Model file for the job. Use its own axes, mm. Give positions to 0.01 mm unless a question says otherwise; leave off trailing zeros. Write each loop counter-clockwise with the first axis right and the second up, starting at its lowest first coordinate (ties: lowest second). Pieces come first, ordered by that corner, then holes. Notation, with made-up numbers: M -7.5,43 L 28.5,43 A16 cw 28.5,67 Z; hole C -10.5,-19.5 d9. An arc over 180 degrees is marked long. Answer as a JSON object with one key per item and string values. Group by question number.
```python
from build123d import *

# Parameters (mm, degrees)
EXTRUSION1_DEPTH      = 5
TROU_TARAUD_M3X0_51_D = 3.3
TROU_TARAUD_M4X0_71_D = 3.3


with BuildPart() as part:
    # Esquisse1 → Extrusion1 (new body)
    with BuildSketch(Plane.XY):
        with BuildLine():
            Line((11.324751653, -14), (-91.324751653, -14))
            ThreePointArc((-91.324751653, -14), (-92.063300599, -13.858640755), (-92.697448823, -13.454545455))
            ThreePointArc((-92.697448823, -13.454545455), (-98.5, 0), (-92.697448823, 13.454545455))
            ThreePointArc((-92.697448823, 13.454545455), (-92.063300599, 13.858640755), (-91.324751653, 14))
            Line((-91.324751653, 14), (11.324751653, 14))
            ThreePointArc((11.324751653, 14), (12.063300599, 13.858640755), (12.697448823, 13.454545455))
            ThreePointArc((12.697448823, 13.454545455), (18.5, 0), (12.697448823, -13.454545455))
            ThreePointArc((12.697448823, -13.454545455), (12.063300599, -13.858640755), (11.324751653, -14))
        make_face()
    extrude(amount=EXTRUSION1_DEPTH)

    # Trou taraudé M3x0.51 (through all)
    with Locations(Plane.XY.offset(5)):
        with Locations((-93.6, -5), (-93.6, 5), (-45.6, -5), (-45.6, 5), (-34.4, -5), (-34.4, 5), (13.6, -5), (13.6, 5)):
            Hole(TROU_TARAUD_M3X0_51_D / 2)

    # Trou taraudé M4x0.71 (through all)
    with Locations(Plane(origin=(0, 0, 0), x_dir=(-1, 0, 0), z_dir=(0, 0, -1))):
        with Locations((0, 0)):
            Hole(TROU_TARAUD_M4X0_71_D / 2)


solid = part.part
```
Q1. Slice it at D-D, the plane x = 0.5. Write the cut outline in (y, z).
Q2. Slice it at B-B, the plane z = 2.2. Count the separate pieces of the cut face and the enclosed holes in it, then the cut area to 3 significant figures.
Q3. Slice it at A-A, the plane x = -45.6. Write the cut outline in (y, z), then the cut area to 3 significant figures.
Q4. Drop flat-ended pins along their axis: P1, Ø3, axis at x = -34.4, y = 5, coming from the +Z side; P2, Ø3, axis at y = 2, z = 2.5, coming from the -X side; P3, Ø1, axis at y = 9.5, z = 4, coming from the +X side; P4, Ø2, axis at y = -2.5, z = 1.5, coming from the -X side. Give the stop position or say it passes through.
Q5. Wall check: L1, parallel to X at y = -5.5, z = 3.6; L2, parallel to Y at x = -45.6, z = 1.6; L3, parallel to X at y = 6.5, z = 4.15. Give the ranges that are in metal, low to high.
Q6. Two-plate mould, pull along Y, no slides. Class faces 1 (the cylindrical face through (14, 3.4, 2.5)), 2 (the cylindrical face through (-98.5, -0.2, 2.5)), 3 (the flat face through (-41, 14, 2)), 4 (the cylindrical face through (15.25, -4.93, 2.47)): +Y half, -Y half, draft (parallel to the pull), parting line (faces both ways), or undercut.
Q7. Slice it at C-C, the plane y = 5. Write the cut outline in (x, z), then the cut area to 3 significant figures.
Solved:
{
 "1": {"outline": "M -14,0 L -1.57,0 L -1.57,5 L -14,5 Z; M 1.57,0 L 14,0 L 14,5 L 1.57,5 Z"},
 "2": {"separate pieces": "1", "enclosed holes": "9", "area": "3,090 mm²"},
 "3": {"outline": "M -14,0 L -6.65,0 L -6.65,5 L -14,5 Z; M -3.35,0 L 3.35,0 L 3.35,5 L -3.35,5 Z; M 6.65,0 L 14,0 L 14,5 L 6.65,5 Z", "area": "107 mm²"},
 "4": {"P1": "passes through", "P2": "stops at x = -98.49", "P3": "stops at x = 16.16", "P4": "stops at x = -98.44"},
 "5": {"L1": "x = -97.66 to -95.17, -92.03 to -47.17, -44.03 to -35.97, -32.83 to 12.03, 15.17 to 17.66", "L2": "y = -14 to -6.65, -3.35 to 3.35, 6.65 to 14", "L3": "x = -97.32 to -94.29, -92.91 to -46.29, -44.91 to -35.09, -33.71 to 12.91, 14.29 to 17.32"},
 "6": {"face 1": "undercut", "face 2": "parting line", "face 3": "+Y half", "face 4": "undercut"},
 "7": {"outline": "M -97.81,0 L -95.25,0 L -95.25,5 L -97.81,5 Z; M -91.95,0 L -47.25,0 L -47.25,5 L -91.95,5 Z; M -43.95,0 L -36.05,0 L -36.05,5 L -43.95,5 Z; M -32.75,0 L 11.95,0 L 11.95,5 L -32.75,5 Z; M 15.25,0 L 17.81,0 L 17.81,5 L 15.25,5 Z", "area": "512 mm²"}
}
